from build123d import *

# Parameters (mm, degrees)
F0_W     = 1.27
F0_H     = 44.45
F0_W_2   = 6.35
F1_DEPTH = 63.5
F2_W     = 105.41
F2_H     = 46.99
F3_DEPTH = 1.27
F4_R     = 3.17


with BuildPart() as f1:
    # F0 (on Top) → F1 (new body)
    with BuildSketch(Plane.XY):
        Polygon((19.05, -22.225), (12.7, -22.225), (-12.7, -22.225), (-12.7, 22.225), (-13.97, 22.225), (-13.97, -22.225), (-13.97, -23.495), (91.44, -23.495), (91.44, -22.225), (90.17, -22.225), (73.66, -22.225), (67.31, -22.225), (50.8, -22.225), (44.45, -22.225), align=None)
        Polygon((-12.7, 22.225), (12.7, 22.225), (19.05, 22.225), (44.45, 22.225), (50.8, 22.225), (67.31, 22.225), (73.66, 22.225), (90.17, 22.225), (91.44, 22.225), (91.44, 23.495), (-13.97, 23.495), (-13.97, 22.225), align=None)
        with Locations((90.805, 0)):
            Rectangle(F0_W, F0_H)
        Polygon((67.31, 22.225), (67.31, -22.225), (73.66, -22.225), (73.66, 0), (73.66, 22.225), align=None)
        with Locations((47.625, 0)):
            Rectangle(F0_W_2, F0_H)
        with Locations((15.875, 0)):
            Rectangle(F0_W_2, F0_H)
    extrude(amount=-F1_DEPTH)

    # F2 (on face) → F3 (join)
    with BuildSketch(Plane(origin=(0, 0, -63.5), x_dir=(1, 0, 0), z_dir=(0, 0, -1))):
        with Locations((38.735, 0)):
            Rectangle(F2_W, F2_H)
    extrude(amount=F3_DEPTH)

    # F4
    f4_edges = [f1.edges().sort_by_distance(p)[0] for p in [
        (19.05, 0, 0),
        (12.7, 0, 0),
        (44.45, 0, 0),
        (50.8, 0, 0),
        (67.31, 0, 0),
        (73.66, 0, 0),
    ]]
    fillet(f4_edges, radius=F4_R)


solid = f1.part
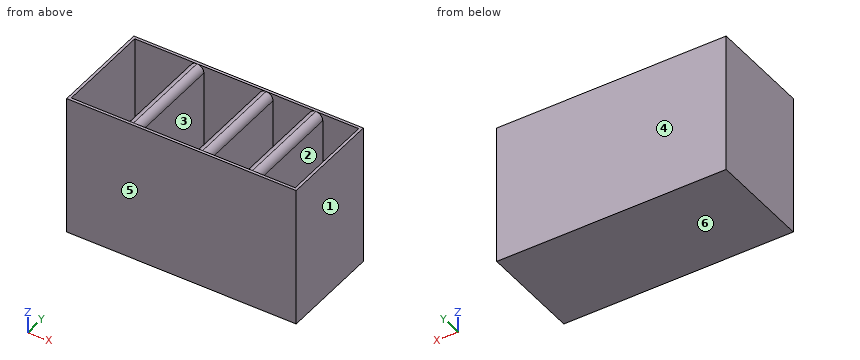
Could you check a few things on this model? Use its own coordinates, in mm. Face numbers are marked on the shaded views. A direction names the side the tool comes from. Round coordinates to 2 decimals unless told otherwise and drop trailing zeros. Order: outer loops, then holes, each group sorted by start corner. A loop starts at its lowest first (then second) coordinate and runs counter-clockwise, first axis right, second up. Notation, with made-up numbers: M 54,-24.5 L 60,-24.5 A23 ccw 60,9.5 Z; hole C 82.25,-23.5 d10. An arc over 180 degrees is marked long. One line per item, written item: value.
(1) Imagine slicing it at B-B (x = 53). Write out the boundary of the cut face in (y, z) (3 decimals).
Ans:
outline: M -23.495,-64.77 L 23.495,-64.77 L 23.495,0 L 22.225,0 L 22.225,-63.5 L -22.225,-63.5 L -22.225,0 L -23.495,0 Z
(2) If we mould it in two halves opening along Y, with no side actions, what happens to the marked faces 3, 4, 5 and 6? For each: released by +Y, released by -Y, zero draft, split by the parting line, or undercut.
Ans:
face 3: undercut
face 4: released by +Y
face 5: released by -Y
face 6: zero draft
(3) I need wall thicknesses on line 1 along X through (y, z) = (18, -5); line 2 along Y through (x, z) = (-7.5, -61.5) (3 decimals). Which ranges of each line are inside material? Lowest first, please. Write a range as from..to.
Ans:
line 1: x = -13.97..-12.7, 12.7..19.05, 44.45..50.8, 67.31..73.66, 90.17..91.44
line 2: y = -23.495..-22.225, 22.225..23.495
(4) I'm going to push a flat-ended pin straight in: P1, Ø13, axis at x = 58.5, y = -2, coming from the +Z side. Where does the tip first touch, or does it pass through?
Ans:
P1: stops at z = -63.5
(5) Imagine slicing it at A-A (z = -22). Write out the boundary of the cut face in (x, y) (3 decimals).
Ans:
outline: M -13.97,-23.495 L 91.44,-23.495 L 91.44,23.495 L -13.97,23.495 Z; hole M -12.7,-22.225 L 12.7,-22.225 L 12.7,22.225 L -12.7,22.225 Z; hole M 19.05,-22.225 L 44.45,-22.225 L 44.45,22.225 L 19.05,22.225 Z; hole M 50.8,-22.225 L 67.31,-22.225 L 67.31,22.225 L 50.8,22.225 Z; hole M 73.66,-22.225 L 90.17,-22.225 L 90.17,22.225 L 73.66,22.225 Z
(6) Which directions (+Z, -Z, +X, -X, +Y, -Y) give clear straight access to the entire face, cutting with the end or side of a thin tool? Please do the marked faces 1 and 2.
Ans:
face 1: +Z, -Z, +X, +Y, -Y
face 2: +Z
